from build123d import *

# Parameters (mm, degrees)
SKETCH1_R           = 4.5
BOSS_EXTRUDE1_DEPTH = 0.3
DOME1_FACE_RADIUS   = 4.5
DOME1_HEIGHT        = 1
SKETCH2_R           = 4
BOSS_EXTRUDE2_DEPTH = 12.5


with BuildPart() as part:
    # Sketch1 → Boss-Extrude1 (new body)
    with BuildSketch(Plane(origin=(0, 0, 0), x_dir=(1, 0, 0), z_dir=(0, 1, 0))):
        with Locations(Location((0, 0, 0), (0, 0, 270))):
            Circle(SKETCH1_R)
    extrude(amount=BOSS_EXTRUDE1_DEPTH)

    # Dome1: a dome of height H over a round flat face of radius A is a cap of a sphere of radius (A * A + H * H) / (2 * H)
    dome1_r = (DOME1_FACE_RADIUS * DOME1_FACE_RADIUS + DOME1_HEIGHT * DOME1_HEIGHT) / (2 * DOME1_HEIGHT)
    dome1_base = Plane((0, 0, 0), z_dir=(0, -1, 0))
    with Locations(dome1_base.offset(DOME1_HEIGHT - dome1_r)):
        dome1_ball = Sphere(dome1_r, mode=Mode.PRIVATE)
    add(split(dome1_ball, bisect_by=dome1_base, keep=Keep.TOP, mode=Mode.PRIVATE))

    # Sketch2 → Boss-Extrude2 (add)
    with BuildSketch(Plane(origin=(0, 0.3, 0), x_dir=(1, 0, 0), z_dir=(0, 1, 0))):
        with Locations(Location((0, 0, 0), (0, 0, 270))):
            Circle(SKETCH2_R)
    extrude(amount=BOSS_EXTRUDE2_DEPTH)


solid = part.part
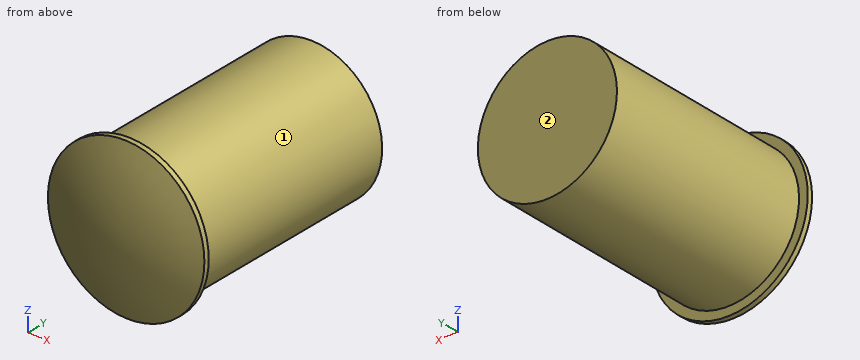
Geometry: final body of the model. Coordinates: model frame, mm. Face numbers are marked on the shaded views. Give positions to 0.01 mm unless a question says otherwise; leave off trailing zeros. Write each loop counter-clockwise with the first axis right and the second up, starting at its lowest first coordinate (ties: lowest second). Pieces come first, ordered by that corner, then holes. Notation, with made-up numbers: (-26, 82) - (-21, 82) arc R29 cw to (-21, 105) - close; hole circle Ø8 at (-21.75, 87). An arc over 180 degrees is marked (long way). Return JSON: item names as keys, results as strings. Group by question number.
1) First-contact query: P1, Ø5, axis at y = 6.5, z = -1.5, coming from the +X side; P2, Ø1, axis at y = 1.5, z = -3, coming from the +X side; P3, Ø4, axis at y = 9.5, z = 0, coming from the -X side. Flat tips, straight axial feed; report the tip coordinate or a pass-through.
2) Section A-A on z = 0. Return the cut outline in (x, y) (3 decimals).
3) Section C-C on y = 8. Return the cut outline in (x, z), plus the area to 3 significant figures.
4) Mould query, pull axis Z, two halves, no side actions, for the marked faces 1 and 2. Classes: released by +Z, released by -Z, zero draft, split by the parting line, or undercut.
5) Section B-B on x = 0. Return the cut outline in (y, z) (3 decimals), plus the area to 3 significant figures.
6) Line query: line 1 (X direction, y = 10.25, z = 3); line 2 (Y direction, x = -0.5, z = 0.25); line 3 (X direction, y = 6, z = -0.5). Output: solid intervals per line, ascending.
Filled in:
{
 "1": {"P1": "stops at x = 4", "P2": "stops at x = 3.12", "P3": "stops at x = -4"},
 "2": {"outline": "(-4.5, 0) arc R10.625 ccw to (4.5, 0) - (4.5, 0.3) - (4, 0.3) - (4, 12.8) - (-4, 12.8) - (-4, 0.3) - (-4.5, 0.3) - close"},
 "3": {"outline": "circle Ø8 at (0, 0)", "area": "50.3 mm^2"},
 "4": {"face 1": "split by the parting line", "face 2": "zero draft"},
 "5": {"outline": "(0, -4.5) - (0.3, -4.5) - (0.3, -4) - (12.8, -4) - (12.8, 4) - (0.3, 4) - (0.3, 4.5) - (0, 4.5) arc R10.625 ccw to start", "area": "109 mm^2"},
 "6": {"line 1": "x = -2.65 to 2.65", "line 2": "y = -0.99 to 12.8", "line 3": "x = -3.97 to 3.97"}
}
